```python
from build123d import *

# Parameters (mm, degrees)
SKETCH1_W           = 12.2
SKETCH1_H           = 22.5
BOSS_EXTRUDE1_DEPTH = 3
FILLET2_R           = 10


with BuildPart() as part:
    # Sketch1 → Boss-Extrude1 (new body)
    with BuildSketch(Plane(origin=(0, 0, 0), x_dir=(1, 0, 0), z_dir=(0, 1, 0))):
        Polygon((-11.1, -16.25), (11.7, -16.25), (11.7, 17.128517662), (-11.1, 17.128517662), (-25, 34.565348469), (-25, 68.106999691), (-29.68539708, 33.799719695), align=None)
        Rectangle(SKETCH1_W, SKETCH1_H, mode=Mode.SUBTRACT)
    extrude(amount=BOSS_EXTRUDE1_DEPTH)

    # Fillet2
    fillet2_edges = [part.edges().sort_by_distance(p)[0] for p in [
        (11.7, 1.5, 16.25),
        (-11.1, 1.5, 16.25),
        (-29.68539708, 1.5, -33.799719695),
        (-25, 1.5, -34.565348469),
        (-11.1, 1.5, -17.128517662),
        (11.7, 1.5, -17.128517662),
    ]]
    fillet(fillet2_edges, radius=FILLET2_R)


solid = part.part
```
CAD build for the part. Positions are in the model's coordinates, mm. A direction names the side the tool comes from. Round coordinates to 2 decimals unless told otherwise and drop trailing zeros. Loops run counter-clockwise (first coordinate to the right, second up) from the corner with the lowest first, then second, coordinate; pieces in that order, holes last. Notation, with made-up numbers: (39.25, -17) - (88.25, -17) arc R30 ccw to (88.25, 21) - close; hole circle Ø10 at (70.5, 40.25). An arc over 180 degrees is marked (long way). Return JSON: item names as keys, results as strings. Group by question number.
Q1. Band-saw the part on D-D on z = -39.5. Give the cut face in (x, y).
Q2. Band-saw the part on C-C on z = 7.5. Give the cut face in (x, y).
Q3. Drill centre lines: line 1 along Z through (x, y) = (-0.5, 0.75); line 2 along X through (y, z) = (2.8, -6.5). Where is each one in solid material? Low to high. Write a range as [from, to].
Q4. Band-saw the part on A-A on x = -3. Give the cut face in (y, z), plus the area to 3 significant figures.
Q5. Band-saw the part on B-B on y = 1.05. Give the cut face in (x, z).
Q6. Two-plate mould, pull along Z, no slides. Class faces 4 (the face through (0, 1, -11.25)), 5 (the face through (-2, 1, -17.129)), 6 (the face through (-9, 3, -11)): +Z half, -Z half, draft (parallel to the pull), parting line (faces both ways), or undercut.
Q7. Flat gauge pins, fed straight in: pin 1 Ø0.9 at (y, z) = (2, -4.5) entering from -X; pin 2 Ø0.9 at (x, y) = (2.5, 1) entering from -Z; pin 3 Ø1.5 at (y, z) = (1, -47.5) entering from +X; pin 4 Ø8 at (x, z) = (-24, -5.5) entering from -Y. Where does each tip first touch, or does it go through?
Q8. Tool access for faces 1 (the face through (-25, 1, -53)), 2 (the face through (-6.1, 1, 0)), 3 (the face through (-1, 1, 16.25)): list every direction of +Z, -Z, +X, -X, +Y, -Y with a clear straight run to the whole face (end or side of a thin tool).
Solutions:
{
 "1": {"outline": "(-28.91, 0) - (-25, 0) - (-25, 3) - (-28.91, 3) - close"},
 "2": {"outline": "(-14.35, 0) - (-6.1, 0) - (-6.1, 3) - (-14.35, 3) - close; (6.1, 0) - (11.62, 0) - (11.62, 3) - (6.1, 3) - close"},
 "3": {"line 1": "z = [-17.13, -11.25], [11.25, 16.25]", "line 2": "x = [-19.55, -6.1], [6.1, 11.7]"},
 "4": {"outline": "(0, -17.13) - (3, -17.13) - (3, -11.25) - (0, -11.25) - close; (0, 11.25) - (3, 11.25) - (3, 16.25) - (0, 16.25) - close", "area": "32.6 mm^2"},
 "5": {"outline": "(-29.35, -36.28) - (-25, -68.11) - (-25, -38.06) arc R10 cw to (-22.82, -31.83) - (-14.1, -20.9) arc R10 cw to (-6.28, -17.13) - (1.7, -17.13) arc R10 ccw to (11.7, -7.13) - (11.7, 6.25) arc R10 ccw to (1.7, 16.25) - (-4.15, 16.25) arc R10 ccw to (-13.52, 9.73) - (-28.81, -31.45) arc R10 ccw to start; hole (-6.1, -11.25) - (6.1, -11.25) - (6.1, 11.25) - (-6.1, 11.25) - close"},
 "6": {"face 4": "undercut", "face 5": "-Z half", "face 6": "draft"},
 "7": {"pin 1": "stops at x = -18.97", "pin 2": "stops at z = -17.12", "pin 3": "stops at x = -25", "pin 4": "passes through"},
 "8": {"face 1": "-Z, +X, +Y, -Y", "face 2": "+Y, -Y", "face 3": "+Z, +X, -X, +Y, -Y"}
}
